Check sheet for the modelled part. Datum: model origin and axes. Units: mm. Face numbers are marked on the shaded views. A direction names the side the tool comes from. Coordinates: 2 decimals unless noted, no trailing zeros. Loops run counter-clockwise (first coordinate to the right, second up) from the corner with the lowest first, then second, coordinate; pieces in that order, holes last. Notation, with made-up numbers: (89, 77) - (102, 77) arc R25 ccw to (102, 106) - close; hole circle Ø2 at (12, -33). An arc over 180 degrees is marked (long way). Write each question's results on one line, items separated by ' | '. Start each with the question number.
1. Cross-section at B-B (z = 0). Record the cut outline in (x, y), and give its area (3 significant figures).
2. Thickness scan on line 1 (X direction, y = 29.5, z = 3.5); line 2 (X direction, y = 13, z = 65.5); line 3 (Z direction, x = 0, y = 7.5). Record the ranges inside material, lowest first. Write a range as [from, to].
3. Gauge pin test, flat ends, axial feed: P1, Ø8, axis at x = -53, y = 26, coming from the +Z side; P2, Ø8, axis at x = 91.5, y = 3.5, coming from the +Z side; P3, Ø12, axis at x = -89.5, y = 18, coming from the +Z side. Record the tip position at first contact, or that the pin passes through.
4. Cross-section at A-A (x = 0). Record the cut outline in (y, z), and give its area (3 significant figures).
5. Cross-section at D-D (x = -205). Record the cut outline in (y, z), and give its area (3 significant figures).
6. Cross-section at C-C (y = 25). Record the cut outline in (x, z) (1 decimal).
7. Tool access check on the marked faces 1 and 2. Record the directions out of +Z, -Z, +X, -X, +Y, -Y that give a thin tool (end or side, any length) a straight path to the whole face; none if there is none.
Autodesk Inventor part; units mm, degrees
ref_plane "YZ Plane" through (0, 0, 0) normal (1, 0, 0) x (0, 1, 0)
ref_plane "XZ Plane" through (0, 0, 0) normal (0, 1, 0) x (-1, 0, 0)
ref_plane "XY Plane" through (0, 0, 0) normal (0, 0, 1) x (1, 0, 0)
sketch "Flange Sketch" plane through (0, 0, 0) normal (0, 1, 0) x (-1, 0, 0)
  circle A0 centre (0, 0) radius 241.3
  circle A1 centre (0, 0) radius 163.576
  circle A2 centre (0, 0) radius 215.9 construction
  line L0 (0, 0) -> (-55.879, -208.5434) construction
  line L1 (0, 0) -> (0, -215.9) construction
  circle A3 centre (0, 0) radius 182.5625
  dimension "outerDiam" = 482.6
  dimension "innerDiam" = 327.152
  dimension "boltCircle" = 431.8
  dimension "boltOffsetAngle" = 15
  dimension "dimensionE" = 365.125
extrude "Flange Extrusion" add sketch "Flange Sketch" along normal blind 17.4752 contours A0 | A3
extrude "Flange Exrusion2" add sketch "Flange Sketch" along normal blind 31.75 contours A3
hole "Bolt Hole" at (55.879, 0, -208.5434) direction (0, 1, 0) diameter 25.4 depth 17.4752
pattern_circular "Bolt Hole Pattern" count 12 over 360 about axis through (0, -10, 0) along (0, 1, 0) of "Bolt Hole"
equation "\"nominalSize\" = 304.8"
properties part number "AWWA C207-18 Class B Ring and Blind Flange"
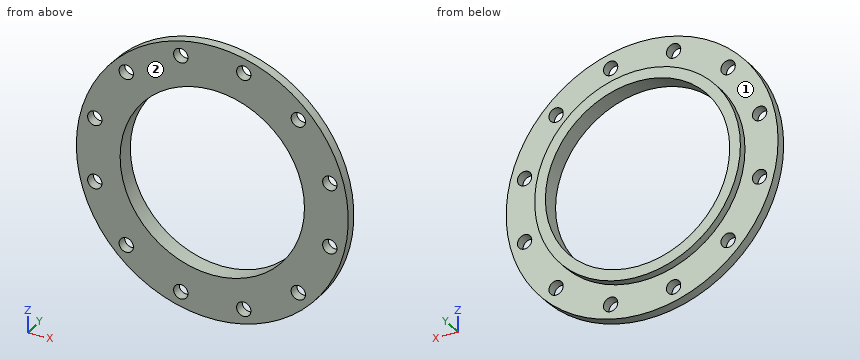
Established:
1) outline: (-241.3, 0) - (-163.58, 0) - (-163.58, 31.75) - (-182.56, 31.75) - (-182.56, 17.48) - (-241.3, 17.48) - close; (163.58, 0) - (241.3, 0) - (241.3, 17.48) - (182.56, 17.48) - (182.56, 31.75) - (163.58, 31.75) - close | area: 3,260 mm^2
2) line 1: [-182.53, -163.54], [163.54, 182.53] | line 2: [-232.24, -216.83], [-200.25, -149.89], [149.89, 200.25], [216.83, 232.24] | line 3: [-241.3, -163.58], [163.58, 241.3]
3) P1: z = 175.86 | P2: z = 224.88 | P3: z = 226.38
4) outline: (0, -241.3) - (17.48, -241.3) - (17.48, -182.56) - (31.75, -182.56) - (31.75, -163.58) - (0, -163.58) - close; (0, 163.58) - (31.75, 163.58) - (31.75, 182.56) - (17.48, 182.56) - (17.48, 241.3) - (0, 241.3) - close | area: 3,260 mm^2
5) outline: (0, -127.28) - (17.48, -127.28) - (17.48, -68.07) - (0, -68.07) - close; (0, -43.68) - (17.48, -43.68) - (17.48, 43.68) - (0, 43.68) - close; (0, 68.07) - (17.48, 68.07) - (17.48, 127.28) - (0, 127.28) - close | area: 3,600 mm^2
6) outline: circle Ø365.1 at (0, 0); hole circle Ø327.2 at (0, 0)
7) face 1: +Y | face 2: +Z, -Z, +X, -X, -Y
